from build123d import *

# Parameters (mm, degrees)
PAD_DEPTH       = 13
POCKET_DEPTH    = 1
SKETCH003_R     = 8
POCKET001_DEPTH = 13.001


with BuildPart() as part:
    # Sketch → Pad (new body)
    with BuildSketch(Plane.XY):
        Polygon((0, 0), (0, 100), (160, 100), (160, -100), (0, -100), align=None)
    extrude(amount=PAD_DEPTH)

    # Sketch002 (on Face7 of Pad) → Pocket (cut)
    with BuildSketch(Plane.XY.offset(13)):
        Polygon((0, -100), (0, -71.973152), (160, -100), align=None)
    extrude(amount=-POCKET_DEPTH, mode=Mode.SUBTRACT)

    # Sketch003 (on Face5 of Pocket) → Pocket001 (cut, through all)
    with BuildSketch(Plane.XY.offset(13)):
        with Locations((60, 37.5)):
            Circle(SKETCH003_R)
        with Locations((135, 37.5)):
            Circle(SKETCH003_R)
        with Locations((135, -37.5)):
            Circle(SKETCH003_R)
        with Locations((60, -37.5)):
            Circle(SKETCH003_R)
    extrude(amount=-POCKET001_DEPTH, mode=Mode.SUBTRACT)


solid = part.part
The listing builds one solid part. Answer for the finished solid, in the listing's coordinates (mm). A direction names the side the tool comes from. Give positions to 0.01 mm unless a question says otherwise; leave off trailing zeros. Loops run counter-clockwise (first coordinate to the right, second up) from the corner with the lowest first, then second, coordinate; pieces in that order, holes last. Notation, with made-up numbers: (-30.75, -20) - (-22.75, -20) arc R20 cw to (-22.75, 10) - close; hole circle Ø8 at (60, 55). An arc over 180 degrees is marked (long way). Answer as a JSON object with one key per item and string values.
1. For faces 1 (the flat face through (78.88, -85.79, 12.51)), 2 (the cylindrical face through (142.63, -35.1, 6.59)), determine the directions among +Z, -Z, +X, -X, +Y, -Y from which every point of the face is accessible in a straight line to the end or side of a thin tool.
Determined:
{"face 1": "+Z, -X, -Y", "face 2": "+Z, -Z"}
2. Flat-ended cylindrical pins translate along their axes: pin 1 Ø13 at (x, y) = (60, 37.5) entering from +Z; pin 2 Ø1.5 at (y, z) = (56, 2.5) entering from -X. Find the tip coordinate at first contact, or state that the pin passes through.
Determined:
{"pin 1": "through", "pin 2": "x = 0"}
3. Find the intervals of material crossed by L1, parallel to Y at x = 60, z = 3.25; L2, parallel to X at y = -42, z = 10.75; L3, parallel to Z at x = 8.5, y = -85.5, in increasing order. Write a range as [from, to].
Determined:
{"L1": "[-100, -45.5], [-29.5, 29.5], [45.5, 100]", "L2": "[0, 53.39], [66.61, 128.39], [141.61, 160]", "L3": "[0, 12]"}
4. For a pull along X with two mould halves and no side action, classify faces 3 (the flat face through (81, -100, 6)), 4 (the flat face through (0, 1, 6)), 5 (the cylindrical face through (54.1, 42.9, 6.6)) as pulls with the +X half, pulls with the -X half, needs draft (parallel to the pull), parting line crosses it, or undercut.
Determined:
{"face 3": "needs draft", "face 4": "pulls with the -X half", "face 5": "undercut"}
5. A cutting plane is placed at A-A (y = -37.5). Write down the section's boundary in (x, z).
Determined:
{"outline": "(0, 0) - (52, 0) - (52, 13) - (0, 13) - close; (68, 0) - (127, 0) - (127, 13) - (68, 13) - close; (143, 0) - (160, 0) - (160, 13) - (143, 13) - close"}
6. A cutting plane is placed at D-D (y = -82). Write down the section's boundary in (x, z).
Determined:
{"outline": "(0, 0) - (160, 0) - (160, 13) - (57.24, 13) - (57.24, 12) - (0, 12) - close"}
7. A cutting plane is placed at C-C (x = 134.5). Write down the section's boundary in (y, z), then the cut area to 3 significant figures.
Determined:
{"outline": "(-100, 0) - (-45.48, 0) - (-45.48, 13) - (-95.53, 13) - (-95.53, 12) - (-100, 12) - close; (-29.52, 0) - (29.52, 0) - (29.52, 13) - (-29.52, 13) - close; (45.48, 0) - (100, 0) - (100, 13) - (45.48, 13) - close", "area": "2,180 mm²"}
8. A cutting plane is placed at B-B (z = 4.5). Write down the section's boundary in (x, y).
Determined:
{"outline": "(0, -100) - (160, -100) - (160, 100) - (0, 100) - close; hole circle Ø16 at (60, -37.5); hole circle Ø16 at (60, 37.5); hole circle Ø16 at (135, -37.5); hole circle Ø16 at (135, 37.5)"}
